Part model, mm, in its own coordinate system. Face numbers are marked on the shaded views. A direction names the side the tool comes from. Round coordinates to 2 decimals unless told otherwise and drop trailing zeros. Loops run counter-clockwise (first coordinate to the right, second up) from the corner with the lowest first, then second, coordinate; pieces in that order, holes last. Notation, with made-up numbers: M 15.25,-21 L 44.25,-21 A8 cw 44.25,-16 Z; hole C 58,33 d5. An arc over 180 degrees is marked long. Put each result on its own line as item: value. Start each with the question number.
```python
from build123d import *

# Parameters (mm, degrees)
BASE_FLANGE1_DEPTH                = 4.7625
EDGE_FLANGE2_STRIP_W              = 20.5232
EDGE_FLANGE2_STRIP_H              = 4.7625
EDGE_FLANGE2_STRIP_CUT_DEPTH      = 76.2
EDGE_FLANGE2_DEPTH                = 76.2
F_1_4_START                       = -50.8
F_1_4_CLEARANCE_HOLE3_OUTLINE_R   = 3.2639
F_1_4_CLEARANCE_HOLE3_DEPTH       = 4.7625
F_1_4_START_2                     = -4.7625
F_1_4_CLEARANCE_HOLE3_2_OUTLINE_R = 3.2639
F_1_4_CLEARANCE_HOLE3_2_DEPTH     = 4.7625
CUT_EXTRUDE1_DEPTH                = 94.877507457


# Read off the part's stored shape, not the designer's step: 1/4 Clearance Hole3
# Sheet-metal steps are written as plain solids
with BuildPart() as part:
    # Sketch1 → Base-Flange1 (new body)
    with BuildSketch(Plane.XY):
        with BuildLine():
            Line((0, 0), (0, -50.8))
            Line((0, -50.8), (-76.2, -50.8))
            Line((-76.2, -50.8), (-76.2, 0))
            ThreePointArc((-76.2, 0), (-38.1, 38.1), (0, 0))
        make_face()
    extrude(amount=-BASE_FLANGE1_DEPTH)

    # Edge-Flange2 strip (across the edge) → Edge-Flange2 strip cut (cut)
    with BuildSketch(Plane(origin=(-76.2, -50.8, 0), x_dir=(0, 1, 0), z_dir=(1, 0, 0))):
        with Locations((-4.7625, -2.38125)):
            Rectangle(EDGE_FLANGE2_STRIP_W, EDGE_FLANGE2_STRIP_H)
    extrude(amount=EDGE_FLANGE2_STRIP_CUT_DEPTH, mode=Mode.SUBTRACT)

    # Edge-Flange2 section (across the edge) → Edge-Flange2 (add)
    with BuildSketch(Plane(origin=(-76.2, -50.8, 0), x_dir=(0, 1, 0), z_dir=(1, 0, 0))):
        with BuildLine():
            Line((0, 0.7366), (0, 20.6375))
            Line((0, 20.6375), (4.7625, 20.6375))
            Line((4.7625, 20.6375), (4.7625, 0.7366))
            ThreePointArc((4.7625, 0.7366), (4.978245145, 0.215745145), (5.4991, 0))
            Line((5.4991, 0), (5.4991, -4.7625))
            ThreePointArc((5.4991, -4.7625), (1.6106491, -3.1518509), (0, 0.7366))
        make_face()
    extrude(amount=EDGE_FLANGE2_DEPTH)

    # 1/4 Clearance Hole3 outline → 1/4 Clearance Hole3 (cut)
    with BuildSketch(Plane(origin=(0, 0, 0), x_dir=(1, 0, 0), z_dir=(0, 1, 0)).offset(F_1_4_START)):
        with Locations((-12.7, -7.9375)):
            Circle(F_1_4_CLEARANCE_HOLE3_OUTLINE_R)
        with Locations((-63.5, -7.9375)):
            Circle(F_1_4_CLEARANCE_HOLE3_OUTLINE_R)
    extrude(amount=F_1_4_CLEARANCE_HOLE3_DEPTH, mode=Mode.SUBTRACT)

    # 1_4 Clearance Hole3 2 outline → 1_4 Clearance Hole3 2 (cut)
    with BuildSketch(Plane.XY.offset(F_1_4_START_2)):
        with Locations((-38.1, 0)):
            Circle(F_1_4_CLEARANCE_HOLE3_2_OUTLINE_R)
    extrude(amount=F_1_4_CLEARANCE_HOLE3_2_DEPTH, mode=Mode.SUBTRACT)

    # Sketch25 → Cut-Extrude1 (cut, through all)
    with BuildSketch(Plane.XY):
        with BuildLine():
            ThreePointArc((-64.811855715, -10.149255602), (-38.48848332, -28.57235912), (-11.673955742, -10.871743644))
            ThreePointArc((-11.673955742, -10.871743644), (-13.402211365, -6.727544988), (-17.546410021, -8.455800612))
            ThreePointArc((-17.546410021, -8.455800612), (-38.402153693, -22.222945983), (-58.875887778, -7.893865468))
            ThreePointArc((-58.875887778, -7.893865468), (-62.971566813, -6.053576567), (-64.811855715, -10.149255602))
        make_face()
    extrude(amount=-CUT_EXTRUDE1_DEPTH, mode=Mode.SUBTRACT)


solid = part.part
```
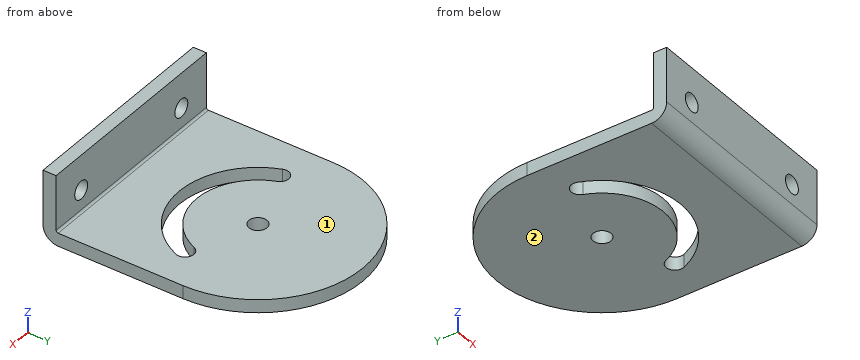
1. Drop flat-ended pins along their axis: pin 1 (10 mm diameter, centred on x = -67.5, y = -32.5, fed in from +Z); pin 2 (4 mm diameter, centred on x = -19, z = 11.5, fed in from +Y). Give the stop position or say it passes through.
2. Which spindle directions (+Z, -Z, +X, -X, +Y, -Y) get a long thin tool onto all of the face, cutting with end or side? Do the marked faces 1 and 2. Say none if no direction does.
3. Cut at B-B, the plane z = 6.75. Give the cut face in (x, y), and give its area (3 significant figures).
4. Cut at A-A, the plane x = -38.1. Give the cut face in (y, z) (1 decimal).
5. Cut at D-D, the plane x = -63.5. Give the cut face in (y, z).
6. Wall check: L1, parallel to Z at x = -40.5, y = -10.5; L2, parallel to Y at x = -55.5, z = 9; L3, parallel to Z at x = -12.7, y = -48.75. Give the ranges that are in metal, low to high.
7. Cut at C-C, the plane z = 1.75. Give the cut face in (x, y).
Results list:
1. pin 1: stops at z = 0
1. pin 2: stops at y = -46.04
2. face 1: +Z, +X, -X, +Y
2. face 2: -Z, +X, -X, +Y, -Y
3. outline: M -76.2,-50.8 L -66.54,-50.8 L -66.54,-46.04 L -76.2,-46.04 Z; M -60.46,-50.8 L -15.74,-50.8 L -15.74,-46.04 L -60.46,-46.04 Z; M -9.66,-50.8 L 0,-50.8 L 0,-46.04 L -9.66,-46.04 Z
3. area: 305 mm^2
4. outline: M -50.8,0.7 A5.5 ccw -45.3,-4.8 L -28.6,-4.8 L -28.6,0 L -45.3,0 A0.7 cw -46,0.7 L -46,20.6 L -50.8,20.6 Z; M -22.2,-4.8 L -3.3,-4.8 L -3.3,0 L -22.2,0 Z; M 3.3,-4.8 L 38.1,-4.8 L 38.1,0 L 3.3,0 Z
5. outline: M -50.8,0.74 A5.5 ccw -45.3,-4.76 L -13.09,-4.76 L -13.09,0 L -45.3,0 A0.74 cw -46.04,0.74 L -46.04,4.67 L -50.8,4.67 Z; M -50.8,11.2 L -46.04,11.2 L -46.04,20.64 L -50.8,20.64 Z; M -6.31,-4.76 L 28.4,-4.76 L 28.4,0 L -6.31,0 Z
6. L1: z = -4.76 to 0
6. L2: y = -50.8 to -46.04
6. L3: z = -3.55 to 4.67, 11.2 to 20.64
7. outline: M -76.2,-50.8 L 0,-50.8 L 0,-46.04 L -76.2,-46.04 Z
